For this review, take the finished solid that the model builds, in its own axes (mm). Face numbers are marked on the shaded views. Coordinates: 2 decimals unless noted, no trailing zeros. Order: outer loops, then holes, each group sorted by start corner. A loop starts at its lowest first (then second) coordinate and runs counter-clockwise, first axis right, second up.
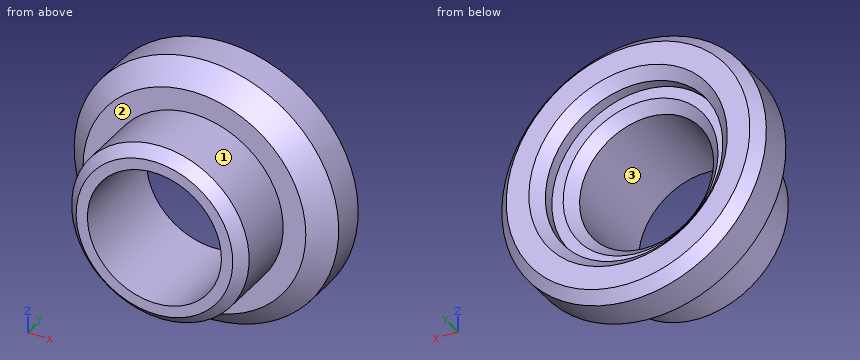
from build123d import *

# Parameters (mm, degrees)
SKETCH1_R           = 9.652
SKETCH1_R_2         = 6.477
BOSS_EXTRUDE1_DEPTH = 3.175
BOSS_EXTRUDE2_START = 3.175
SKETCH1_3_R         = 9.652
SKETCH1_3_R_2       = 6.477
BOSS_EXTRUDE2_DEPTH = 1.5875
BOSS_EXTRUDE3_START = 5.08
SKETCH2_R           = 6.477
SKETCH2_R_2         = 4.8895
BOSS_EXTRUDE3_DEPTH = 5.08
SKETCH3_R           = 4.8895
CUT_EXTRUDE1_DEPTH  = 15.564635526
CHAMFER1_SIZE       = 1.524
CHAMFER2_SIZE       = 0.762
CHAMFER3_SIZE       = 0.762


with BuildPart() as part:
    # Sketch1 → Boss-Extrude1 (new body)
    # profile 1 of 2: a face of its own
    with BuildSketch(Plane(origin=(0, 0, 0), x_dir=(1, 0, 0), z_dir=(0, 1, 0))):
        with Locations(Location((0, 0, 0), (0, 0, 270))):
            Circle(SKETCH1_R)
        Circle(SKETCH1_R_2, mode=Mode.SUBTRACT)
    # profile 2 of 2: a face of its own
    with BuildSketch(Plane(origin=(0, 0, 0), x_dir=(1, 0, 0), z_dir=(0, 1, 0))):
        Circle(SKETCH1_R_2)
    extrude(amount=BOSS_EXTRUDE1_DEPTH)

    # Sketch1<3> → Boss-Extrude2 (add)
    with BuildSketch(Plane(origin=(0, 0, 0), x_dir=(1, 0, 0), z_dir=(0, 1, 0)).offset(BOSS_EXTRUDE2_START)):
        with Locations(Location((0, 0, 0), (0, 0, 270))):
            Circle(SKETCH1_3_R)
        with Locations(Location((0, 0, 0), (0, 0, 270))):
            Circle(SKETCH1_3_R_2, mode=Mode.SUBTRACT)
    extrude(amount=BOSS_EXTRUDE2_DEPTH)

    # Sketch2 → Boss-Extrude3 (add)
    with BuildSketch(Plane.XZ.offset(BOSS_EXTRUDE3_START)):
        with Locations(Location((0, 0, 0), (0, 0, 90))):
            Circle(SKETCH2_R)
        with Locations(Location((0, 0, 0), (0, 0, 270))):
            Circle(SKETCH2_R_2, mode=Mode.SUBTRACT)
    extrude(amount=-BOSS_EXTRUDE3_DEPTH)

    # Sketch3 → Cut-Extrude1 (cut, through all)
    with BuildSketch(Plane.XZ):
        with Locations(Location((0, 0, 0), (0, 0, 90))):
            Circle(SKETCH3_R)
    extrude(amount=-CUT_EXTRUDE1_DEPTH, mode=Mode.SUBTRACT)

    # Chamfer1
    chamfer1_edges = [part.edges().sort_by_distance(p)[0] for p in [
        (0, 0, -9.652),
    ]]
    chamfer(chamfer1_edges, length=CHAMFER1_SIZE)

    # Chamfer2
    chamfer2_edges = [part.edges().sort_by_distance(p)[0] for p in [
        (0, 3.175, -4.8895),
        (0, 4.7625, -9.652),
        (0, 4.7625, -6.477),
    ]]
    chamfer(chamfer2_edges, length=CHAMFER2_SIZE)

    # Chamfer3
    chamfer3_edges = [part.edges().sort_by_distance(p)[0] for p in [
        (0, -5.08, -6.477),
    ]]
    chamfer(chamfer3_edges, length=CHAMFER3_SIZE)


solid = part.part
1. The part is to be moulded in two halves that separate along X. For the marked faces 1, 2 and 3, say which applies: +X half, -X half, draft (parallel to the pull), parting line (faces both ways), or undercut.
Answer below:
face 1: parting line
face 2: draft
face 3: undercut
2. To check wall thickness, follow L1, parallel to X at y = 3.6, z = 0; L2, parallel to X at y = -1, z = 0; L3, parallel to Z at x = 2, y = -2. State the ranges of each line that lie inside material, in increasing order.
Answer below:
L1: x = -9.65 to -6.48, 6.48 to 9.65
L2: x = -6.48 to -4.89, 4.89 to 6.48
L3: z = -6.16 to -4.46, 4.46 to 6.16
3. Take a section at B-B, the plane x = 0. Give the boundary of the cut face in (y, z) (1 decimal), plus the area to 3 significant figures.
Answer below:
outline: (-5.1, -5.7) - (-4.3, -6.5) - (0, -6.5) - (0, -8.1) - (1.5, -9.7) - (4, -9.7) - (4.8, -8.9) - (4.8, -7.2) - (4, -6.5) - (3.2, -6.5) - (3.2, -5.7) - (2.4, -4.9) - (-5.1, -4.9) - close; (-5.1, 4.9) - (2.4, 4.9) - (3.2, 5.7) - (3.2, 6.5) - (4, 6.5) - (4.8, 7.2) - (4.8, 8.9) - (4, 9.7) - (1.5, 9.7) - (0, 8.1) - (0, 6.5) - (-4.3, 6.5) - (-5.1, 5.7) - close
area: 51.8 mm2
4. Clearance check with flat-ended pins moving along their axes: pin 1 Ø1 at (y, z) = (1.5, 3.5) entering from -X; pin 2 Ø1 at (x, y) = (3, -1) entering from -Z; pin 3 Ø4 at (x, z) = (-1, -1) entering from +Y; pin 4 Ø3 at (x, y) = (-3.5, -1) entering from +Z. State where each tip first meets the part, or that it passes through.
Answer below:
pin 1: stops at x = -9.17
pin 2: stops at z = -5.98
pin 3: passes through
pin 4: stops at z = 8
5. Take a section at C-C, the plane y = -2. Give the boundary of the cut face in (x, z), plus the area to 3 significant figures.
Answer below:
outline: circle Ø12.95 at (0, 0); hole circle Ø9.78 at (0, 0)
area: 56.7 mm2
6. Take a section at A-A, the plane z = 0. Give the boundary of the cut face in (x, y) (1 decimal).
Answer below:
outline: (-9.7, 1.5) - (-8.1, 0) - (-6.5, 0) - (-6.5, -4.3) - (-5.7, -5.1) - (-4.9, -5.1) - (-4.9, 2.4) - (-5.7, 3.2) - (-6.5, 3.2) - (-6.5, 4) - (-7.2, 4.8) - (-8.9, 4.8) - (-9.7, 4) - close; (4.9, -5.1) - (5.7, -5.1) - (6.5, -4.3) - (6.5, 0) - (8.1, 0) - (9.7, 1.5) - (9.7, 4) - (8.9, 4.8) - (7.2, 4.8) - (6.5, 4) - (6.5, 3.2) - (5.7, 3.2) - (4.9, 2.4) - close
